CAD build for the part. Positions are in the model's coordinates, mm. Round coordinates to 2 decimals unless told otherwise and drop trailing zeros. Order: outer loops, then holes, each group sorted by start corner. A loop starts at its lowest first (then second) coordinate and runs counter-clockwise, first axis right, second up. Notation, with made-up numbers: (28.25, 15) - (59.25, 15) arc R20 cw to (59.25, 45) - close; hole circle Ø2 at (-18.75, -37.75). An arc over 180 degrees is marked (long way). Write item = value, one per line.
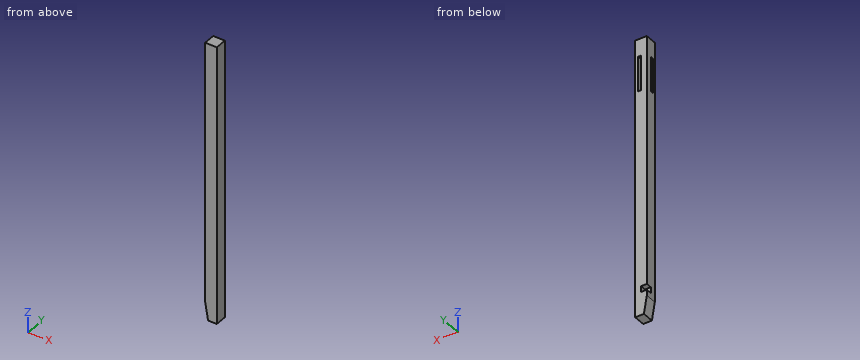
from build123d import *

# Parameters (mm, degrees)
F0_W     = 25.4
F0_H     = 609.6
F1_DEPTH = 25.4
F3_DEPTH = 25.4
F4_W     = 12.7
F4_H     = 12.7
F5_DEPTH = 12.7
F6_W     = 6.35
F6_H     = 76.2
F7_DEPTH = 12.7
F8_W     = 6.35
F8_H     = 76.2
F9_DEPTH = 12.446


with BuildPart() as f1:
    # F0 (on Front) → F1 (new body)
    with BuildSketch(Plane.XZ):
        Rectangle(F0_W, F0_H)
    extrude(amount=F1_DEPTH)

    # F2 (on face) → F3 (cut)
    with BuildSketch(Plane.XZ.offset(25.4)):
        Polygon((-12.7, -304.8), (-6.35, -304.8), (-12.7, -266.7), align=None)
    extrude(amount=-F3_DEPTH, mode=Mode.SUBTRACT)

    # F4 (on face) → F5 (cut)
    with BuildSketch(Plane(origin=(-12.7, 0, 0), x_dir=(0, -1, 0), z_dir=(-1, 0, 0))):
        with Locations((6.35, -247.65)):
            Rectangle(F4_W, F4_H)
    extrude(amount=-F5_DEPTH, mode=Mode.SUBTRACT)

    # F6 (on face) → F7 (cut)
    with BuildSketch(Plane(origin=(-12.7, 0, 0), x_dir=(0, -1, 0), z_dir=(-1, 0, 0))):
        with Locations((15.875, 228.6)):
            Rectangle(F6_W, F6_H)
    extrude(amount=-F7_DEPTH, mode=Mode.SUBTRACT)

    # F8 (on face) → F9 (cut)
    with BuildSketch(Plane(origin=(0, 0, 0), x_dir=(-1, 0, 0), z_dir=(0, 1, 0))):
        with Locations((-3.175, 228.6)):
            Rectangle(F8_W, F8_H)
    extrude(amount=-F9_DEPTH, mode=Mode.SUBTRACT)


solid = f1.part
(1) Band-saw the part on A-A on y = -7.5. List the corners of the cut face in (x, z).
Solved:
outline = (-12.7, -266.7) - (-6.35, -304.8) - (12.7, -304.8) - (12.7, 304.8) - (-12.7, 304.8) - (-12.7, -241.3) - (0, -241.3) - (0, -254) - (-12.7, -254) - close; hole (0, 190.5) - (6.35, 190.5) - (6.35, 266.7) - (0, 266.7) - close
(2) Drop flat-ended pins along their axis: pin 1 (10 mm diameter, centred on y = -15.5, z = 217.5, fed in from -X); pin 2 (4 mm diameter, centred on y = -7, z = -246, fed in from -X). Give the stop position or say it passes through.
Solved:
pin_1 = -12.7
pin_2 = 0
(3) Probe line 1 along Z through (x, y) = (-4.25, -1); line 2 along X through (y, z) = (-5.5, 238.5); line 3 along Z through (x, y) = (3.5, -12). List the from-to ranges inside material, lowest first.
Solved:
line_1 = -304.8 to -254, -241.3 to 304.8
line_2 = -12.7 to 0, 6.35 to 12.7
line_3 = -304.8 to 190.5, 266.7 to 304.8
